from build123d import *

# Parameters (mm, degrees)
SKETCH1_W           = 2
SKETCH1_H           = 2
BOSS_EXTRUDE1_DEPTH = 15
SKETCH4_W           = 2
SKETCH4_H           = 2
BOSS_EXTRUDE3_DEPTH = 15
SKETCH5_W           = 2
SKETCH5_H           = 2
BOSS_EXTRUDE4_DEPTH = 11
SKETCH6_W           = 38
SKETCH6_H           = 8
BOSS_EXTRUDE5_DEPTH = 2
SKETCH8_W           = 4
SKETCH8_H           = 5
BOSS_EXTRUDE6_DEPTH = 2
SKETCH9_W           = 4
SKETCH9_H           = 5
BOSS_EXTRUDE7_DEPTH = 2
SKETCH10_W          = 2
SKETCH10_H          = 5
BOSS_EXTRUDE8_DEPTH = 2
SKETCH11_W          = 2
SKETCH11_H          = 5
BOSS_EXTRUDE9_DEPTH = 2


with BuildPart() as part:
    # Sketch1 → Boss-Extrude1 (new body)
    with BuildSketch(Plane.XY):
        Rectangle(SKETCH1_W, SKETCH1_H)
    extrude(amount=BOSS_EXTRUDE1_DEPTH)

    # Sketch4 → Boss-Extrude3 (add)
    with BuildSketch(Plane(origin=(1, 0, 0), x_dir=(0, 0, -1), z_dir=(1, 0, 0))):
        with Locations((-1, 0)):
            Rectangle(SKETCH4_W, SKETCH4_H)
    extrude(amount=BOSS_EXTRUDE3_DEPTH)

    # Sketch5 → Boss-Extrude4 (add)
    with BuildSketch(Plane.XY.offset(2)):
        with Locations((15, 0)):
            Rectangle(SKETCH5_W, SKETCH5_H)
    extrude(amount=BOSS_EXTRUDE4_DEPTH)

    # Sketch6 → Boss-Extrude5 (add)
    with BuildSketch(Plane.XY.offset(15)):
        with Locations((13.360084104, 1.19652769)):
            Rectangle(SKETCH6_W, SKETCH6_H)
    extrude(amount=BOSS_EXTRUDE5_DEPTH)

    # Sketch8 → Boss-Extrude6 (add)
    with BuildSketch(Plane(origin=(32.360084104, 0, 0), x_dir=(0, 0, -1), z_dir=(1, 0, 0))):
        with Locations((-19, 0.971825631)):
            Rectangle(SKETCH8_W, SKETCH8_H)
    extrude(amount=-BOSS_EXTRUDE6_DEPTH)

    # Sketch9 → Boss-Extrude7 (add)
    with BuildSketch(Plane.ZY.offset(5.639915896)):
        with Locations((19, 1.508383794)):
            Rectangle(SKETCH9_W, SKETCH9_H)
    extrude(amount=-BOSS_EXTRUDE7_DEPTH)

    # Sketch10 → Boss-Extrude8 (add)
    with BuildSketch(Plane(origin=(-3.639915896, 0, 0), x_dir=(0, 0, -1), z_dir=(1, 0, 0))):
        with Locations((-20, 1.508383794)):
            Rectangle(SKETCH10_W, SKETCH10_H)
    extrude(amount=BOSS_EXTRUDE8_DEPTH)

    # Sketch11 → Boss-Extrude9 (add)
    with BuildSketch(Plane.ZY.offset(-30.360084104)):
        with Locations((20, 0.971825631)):
            Rectangle(SKETCH11_W, SKETCH11_H)
    extrude(amount=BOSS_EXTRUDE9_DEPTH)


solid = part.part
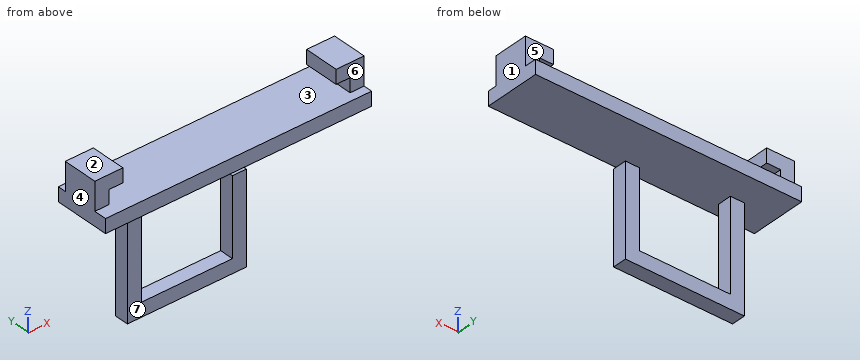
Geometry check sheet. Reference: the model listing, model coordinates, mm. Face numbers are marked on the shaded views. A direction names the side the tool comes from. Round coordinates to 2 decimals unless told otherwise and drop trailing zeros. Order: outer loops, then holes, each group sorted by start corner. A loop starts at its lowest first (then second) coordinate and runs counter-clockwise, first axis right, second up. Notation, with made-up numbers: M -34.75,-7 L -22.75,-7 A26 cw -22.75,8 Z; hole C -3,31 d7. An arc over 180 degrees is marked long. Write each question's results on one line, items separated by ' | '. Start each with the question number.
1. Go/stop test with flat-tipped pins: P1, Ø2, axis at x = -2.5, y = 1.5, coming from the -Z side; P2, Ø7.5, axis at x = 4.5, z = 9, coming from the +Y side; P3, Ø1, axis at y = 0, z = 5, coming from the -X side. Record where each tip stops, or that it passes through.
2. Material ranges on L1, parallel to X at y = 0, z = 9; L2, parallel to X at y = 1.25, z = 20; L3, parallel to Z at x = 13.5, y = 0.5, recorded low to high. Write a range as from..to.
3. Cross-section at A-A on x = 9.5. Record the boundary of the cut face in (y, z), plus the area to 3 significant figures.
4. Cross-section at B-B on z = 4. Record the boundary of the cut face in (x, y).
5. Cross-section at D-D on y = 0.25. Record the boundary of the cut face in (x, z), plus the area to 3 significant figures.
6. Set-up check for the marked faces 5, 6 and 7: record each of +Z, -Z, +X, -X, +Y, -Y from which the full face is reachable in a straight line by a thin tool's end or side.
7. Cross-section at C-C on y = 3. Record the boundary of the cut face in (x, z).
8. Draft check along X on the marked faces 1, 2, 3 and 4. Enter one of: pulls with the +X half, pulls with the -X half, needs draft (parallel to the pull), parting line crosses it, or undercut.
Resolved:
1) P1: z = 15 | P2: y = 1 | P3: x = -1
2) L1: -1..1, 14..16 | L2: -5.64..-1.64, 28.36..32.36 | L3: 0..2, 15..17
3) outline: M -2.8,15 L 5.2,15 L 5.2,17 L -2.8,17 Z; M -1,0 L 1,0 L 1,2 L -1,2 Z | area: 20.0 mm2
4) outline: M -1,-1 L 1,-1 L 1,1 L -1,1 Z; M 14,-1 L 16,-1 L 16,1 L 14,1 Z
5) outline: M -5.64,15 L -1,15 L -1,0 L 16,0 L 16,13 L 14,13 L 14,2 L 1,2 L 1,15 L 32.36,15 L 32.36,21 L 28.36,21 L 28.36,19 L 30.36,19 L 30.36,17 L -3.64,17 L -3.64,19 L -1.64,19 L -1.64,21 L -5.64,21 Z | area: 182 mm2
6) face 5: +Z, +X, +Y | face 6: +Z, +X, -X, -Y | face 7: -Z, +X, -X, -Y
7) outline: M -5.64,15 L 32.36,15 L 32.36,21 L 28.36,21 L 28.36,19 L 30.36,19 L 30.36,17 L -3.64,17 L -3.64,19 L -1.64,19 L -1.64,21 L -5.64,21 Z
8) face 1: pulls with the +X half | face 2: needs draft | face 3: undercut | face 4: pulls with the -X half
